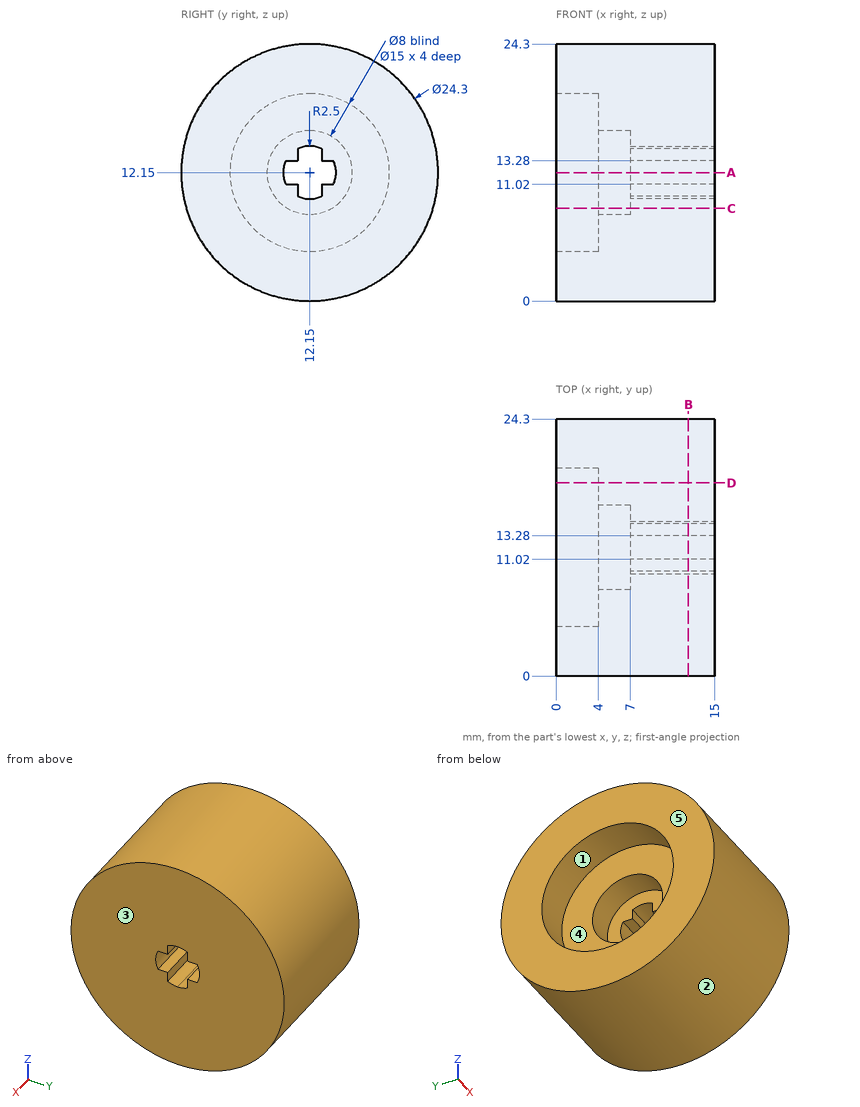
Study the drawing (mm; zero at the part's minimum x, y, z) and answer. A direction names the side the tool comes from. Coordinates: 2 decimals unless noted, no trailing zeros. Write each loop counter-clockwise with the first axis right and the second up, starting at its lowest first coordinate (ties: lowest second). Pieces come first, ordered by that corner, then holes. Notation, with made-up numbers: (14, -10) - (69, -10) arc R24 cw to (69, 4) - close; hole circle Ø8 at (71, -8). An arc over 180 degrees is marked (long way). One line per question, with ' | ' between items.
1) Find section A-A, the plane z = 12.15. Determine the outline of the cut face in (x, y).
Checks:
outline: (0, 0) - (15, 0) - (15, 9.65) - (7, 9.65) - (7, 8.15) - (4, 8.15) - (4, 4.65) - (0, 4.65) - close; (0, 19.65) - (4, 19.65) - (4, 16.15) - (7, 16.15) - (7, 14.65) - (15, 14.65) - (15, 24.3) - (0, 24.3) - close
2) For the marked faces 4 and 5, determine the directions among +Z, -Z, +X, -X, +Y, -Y from which every point of the face is accessible in a straight line to the end or side of a thin tool.
Checks:
face 4: -X | face 5: +Z, -Z, -X, +Y, -Y
3) Consider probe 1 along Y at (x, z) = (1.85, 12.15); probe 2 along Y at (x, z) = (4.95, 12.15); probe 3 along X at (y, z) = (16.25, 17.5). Determine where each line is inside the solid, lowest interval first. Write a range as [from, to].
Checks:
probe 1: [0, 4.65], [19.65, 24.3] | probe 2: [0, 8.15], [16.15, 24.3] | probe 3: [4, 15]
4) Flat-ended cylindrical pins translate along their axes: P1, Ø0.6, axis at x = 12, y = 14, coming from the -Z side; P2, Ø4, axis at x = 8.5, z = 14.5, coming from the +Y side (3 decimals); P3, Ø0.9, axis at x = 12, y = 14, coming from the +Z side. Find the tip coordinate at first contact, or state that the pin passes through.
Checks:
P1: z = 0.1 | P2: y = 24.295 | P3: z = 24.22
5) Find section D-D, the plane y = 18.25. Determine the outline of the cut face in (x, z).
Checks:
outline: (0, 1.64) - (15, 1.64) - (15, 22.66) - (0, 22.66) - (0, 16.51) - (4, 16.51) - (4, 7.79) - (0, 7.79) - close
6) Find section B-B, the plane x = 12.5. Determine the outline of the cut face in (y, z), and give its area (3 significant figures).
Checks:
outline: circle Ø24.3 at (12.15, 12.15); hole (9.92, 11.02) - (11.02, 11.02) - (11.02, 9.92) arc R2.5 ccw to (13.28, 9.92) - (13.28, 11.02) - (14.38, 11.02) arc R2.5 ccw to (14.38, 13.28) - (13.28, 13.28) - (13.28, 14.38) arc R2.5 ccw to (11.02, 14.38) - (11.02, 13.28) - (9.92, 13.28) arc R2.5 ccw to start | area: 447 mm2
7) The mould has two halves that part along Y. Classify the marked faces 1, 2 and 3: +Y half, -Y half, draft (parallel to the pull), parting line (faces both ways), or undercut.
Checks:
face 1: undercut | face 2: parting line | face 3: draft
8) Find section C-C, the plane z = 8.75. Determine the outline of the cut face in (x, y) (3 decimals), and give its area (3 significant figures).
Checks:
outline: (0, 0.485) - (15, 0.485) - (15, 23.815) - (0, 23.815) - (0, 18.835) - (4, 18.835) - (4, 14.257) - (7, 14.257) - (7, 10.043) - (4, 10.043) - (4, 5.465) - (0, 5.465) - close | area: 284 mm2
